Read the model definition and answer for the solid it produces. Units are mm, in the model's axes. Face numbers are marked on the shaded views. A direction names the side the tool comes from. Give positions to 0.01 mm unless a question says otherwise; leave off trailing zeros. Order: outer loops, then holes, each group sorted by start corner. A loop starts at its lowest first (then second) coordinate and runs counter-clockwise, first axis right, second up. Notation, with made-up numbers: (84, 19.25) - (136, 19.25) arc R11 cw to (136, 28.25) - close; hole circle Ø10 at (48.5, 59). An arc over 180 degrees is marked (long way). Use a Markdown table: item, result. Add a question column.
1. Flat-ended cylindrical pins translate along their axes: P1, Ø8, axis at x = -53, z = -9.5, coming from the +Y side; P2, Ø4, axis at x = -22.5, y = 67.5, coming from the +Z side; P3, Ø5, axis at x = -21, y = 29, coming from the +Z side; P4, Ø1.2, axis at y = 86, z = -42.5, coming from the -X side. Find the tip coordinate at first contact, or state that the pin passes through.
2. A cutting plane is placed at A-A on x = -20. Determine the outline of the cut face in (y, z).
3. A cutting plane is placed at B-B on z = 55. Determine the outline of the cut face in (x, y), and give its area (3 significant figures).
4. A cutting plane is placed at C-C on z = -20. Determine the outline of the cut face in (x, y), and give its area (3 significant figures).
5. Consider L1, parallel to X at y = 1, z = 55; L2, parallel to X at y = 100, z = 22; L3, parallel to X at y = 10.5, z = -57. Determine where each line is inside the solid, lowest interval first.
6. Which of the six approach directions +Z, -Z, +X, -X, +Y, -Y give full straight-line access (tool end or side, diameter ignored) to the marked faces 1, 2, 3, 4 and 5?
7. A cutting plane is placed at D-D on y = 44. Determine the outline of the cut face in (x, z).
```python
from build123d import *

# Parameters (mm, degrees)
SKETCH_2_W          = 140
SKETCH_2_H          = 140
EXTRUDE_1_DEPTH     = 4
EXTRUDE_1_2_DEPTH   = 100
EXTRUDE_2_DEPTH     = 2
CUT_EXTRUDE_1_DEPTH = 115.5
SKETCH_6_R          = 6.5
CUT_EXTRUDE_2_DEPTH = 5
FILLET_1_R          = 10
CUT_EXTRUDE_3_REACH = 116


with BuildPart() as part:
    # Эскиз2 → Extrude 1 (new body)
    with BuildSketch(Plane(origin=(0, 0, 0), x_dir=(1, 0, 0), z_dir=(0, 1, 0))):
        Rectangle(SKETCH_2_W, SKETCH_2_H)
    extrude(amount=EXTRUDE_1_DEPTH)

    # Эскиз3 → Extrude 1 2 (add)
    with BuildSketch(Plane(origin=(0, 4, 0), x_dir=(1, 0, 0), z_dir=(0, 1, 0))):
        with BuildLine():
            Line((-40.5, -40), (-40.5, 39))
            ThreePointArc((-40.5, 39), (-40.207106781, 39.707106781), (-39.5, 40))
            Line((-39.5, 40), (39.5, 40))
            ThreePointArc((39.5, 40), (40.207106781, 39.707106781), (40.5, 39))
            Line((40.5, 39), (40.5, -40))
            Line((40.5, -40), (44.5, -40))
            Line((44.5, -40), (44.5, 39))
            ThreePointArc((44.5, 39), (43.035533906, 42.535533906), (39.5, 44))
            Line((39.5, 44), (-39.5, 44))
            ThreePointArc((-39.5, 44), (-43.035533906, 42.535533906), (-44.5, 39))
            Line((-44.5, 39), (-44.5, -40))
            Line((-44.5, -40), (-40.5, -40))
        make_face()
    extrude(amount=EXTRUDE_1_2_DEPTH)

    # Эскиз4 → Бобышка-Вытянуть2 (add, symmetric)
    with BuildSketch(Plane(origin=(0, 0, 0), x_dir=(0, 0, -1), z_dir=(1, 0, 0))):
        Polygon((44, 40.373066959), (65, 4), (44, 4), align=None)
    extrude(amount=EXTRUDE_2_DEPTH, both=True)

    # Эскиз5 → Вырез-Вытянуть1 (cut, through all)
    with BuildSketch(Plane(origin=(44.5, 0, 0), x_dir=(0, 0, -1), z_dir=(1, 0, 0))):
        with BuildLine():
            Line((-15, 92), (-15, 80))
            ThreePointArc((-15, 80), (-20, 75), (-25, 80))
            Line((-25, 80), (-25, 92))
            ThreePointArc((-25, 92), (-20, 97), (-15, 92))
        make_face()
        with BuildLine():
            Line((-15, 28), (-15, 16))
            ThreePointArc((-15, 16), (-20, 11), (-25, 16))
            Line((-25, 16), (-25, 28))
            ThreePointArc((-25, 28), (-20, 33), (-15, 28))
        make_face()
        with BuildLine():
            Line((15, 92), (15, 80))
            ThreePointArc((15, 80), (20, 75), (25, 80))
            Line((25, 80), (25, 92))
            ThreePointArc((25, 92), (20, 97), (15, 92))
        make_face()
        with BuildLine():
            Line((15, 28), (15, 16))
            ThreePointArc((15, 16), (20, 11), (25, 16))
            Line((25, 16), (25, 28))
            ThreePointArc((25, 28), (20, 33), (15, 28))
        make_face()
    extrude(amount=-CUT_EXTRUDE_1_DEPTH, mode=Mode.SUBTRACT)

    # Эскиз6 → Вырез-Вытянуть2 (cut, through all)
    with BuildSketch(Plane(origin=(0, 4, 0), x_dir=(1, 0, 0), z_dir=(0, 1, 0))):
        with Locations(Location((-55, 55, 0), (0, 0, 270))):  # turned: the seam where the file's is
            Circle(SKETCH_6_R)
        with Locations(Location((-55, -55, 0), (0, 0, 270))):  # turned: the seam where the file's is
            Circle(SKETCH_6_R)
        with Locations(Location((55, 55, 0), (0, 0, 270))):  # turned: the seam where the file's is
            Circle(SKETCH_6_R)
        with Locations(Location((55, -55, 0), (0, 0, 270))):  # turned: the seam where the file's is
            Circle(SKETCH_6_R)
    extrude(amount=-CUT_EXTRUDE_2_DEPTH, mode=Mode.SUBTRACT)

    # Скругление1
    fillet_1_edges = [part.edges().sort_by_distance(p)[0] for p in [
        (70, 2, 70),
        (-70, 2, 70),
        (-70, 2, -70),
        (70, 2, -70),
    ]]
    fillet(fillet_1_edges, radius=FILLET_1_R)

    # Эскиз8 → Вырез-Вытянуть3 (cut, up to next)
    with BuildSketch(Plane(origin=(0, 0, -44), x_dir=(-1, 0, 0), z_dir=(0, 0, -1)), mode=Mode.PRIVATE) as cut_extrude_3_sk1:
        with BuildLine():
            Line((-15, 92), (-15, 80))
            ThreePointArc((-15, 80), (-20, 75), (-25, 80))
            Line((-25, 80), (-25, 92))
            ThreePointArc((-25, 92), (-20, 97), (-15, 92))
        make_face()
    cut_extrude_3_tool1 = extrude(cut_extrude_3_sk1.sketch, amount=-CUT_EXTRUDE_3_REACH, mode=Mode.PRIVATE) & part.part
    add(cut_extrude_3_tool1.solids().sort_by_distance((20, 86, -44))[0], mode=Mode.SUBTRACT)
    # Эскиз8 → Вырез-Вытянуть3 (cut, up to next)
    with BuildSketch(Plane(origin=(0, 0, -44), x_dir=(-1, 0, 0), z_dir=(0, 0, -1)), mode=Mode.PRIVATE) as cut_extrude_3_sk2:
        with BuildLine():
            Line((-15, 28), (-15, 16))
            ThreePointArc((-15, 16), (-20, 11), (-25, 16))
            Line((-25, 16), (-25, 28))
            ThreePointArc((-25, 28), (-20, 33), (-15, 28))
        make_face()
    cut_extrude_3_tool2 = extrude(cut_extrude_3_sk2.sketch, amount=-CUT_EXTRUDE_3_REACH, mode=Mode.PRIVATE) & part.part
    add(cut_extrude_3_tool2.solids().sort_by_distance((20, 22, -44))[0], mode=Mode.SUBTRACT)
    # Эскиз8 → Вырез-Вытянуть3 (cut, up to next)
    with BuildSketch(Plane(origin=(0, 0, -44), x_dir=(-1, 0, 0), z_dir=(0, 0, -1)), mode=Mode.PRIVATE) as cut_extrude_3_sk3:
        with BuildLine():
            Line((15, 92), (15, 80))
            ThreePointArc((15, 80), (20, 75), (25, 80))
            Line((25, 80), (25, 92))
            ThreePointArc((25, 92), (20, 97), (15, 92))
        make_face()
    cut_extrude_3_tool3 = extrude(cut_extrude_3_sk3.sketch, amount=-CUT_EXTRUDE_3_REACH, mode=Mode.PRIVATE) & part.part
    add(cut_extrude_3_tool3.solids().sort_by_distance((-20, 86, -44))[0], mode=Mode.SUBTRACT)
    # Эскиз8 → Вырез-Вытянуть3 (cut, up to next)
    with BuildSketch(Plane(origin=(0, 0, -44), x_dir=(-1, 0, 0), z_dir=(0, 0, -1)), mode=Mode.PRIVATE) as cut_extrude_3_sk4:
        with BuildLine():
            Line((15, 28), (15, 16))
            ThreePointArc((15, 16), (20, 11), (25, 16))
            Line((25, 16), (25, 28))
            ThreePointArc((25, 28), (20, 33), (15, 28))
        make_face()
    cut_extrude_3_tool4 = extrude(cut_extrude_3_sk4.sketch, amount=-CUT_EXTRUDE_3_REACH, mode=Mode.PRIVATE) & part.part
    add(cut_extrude_3_tool4.solids().sort_by_distance((-20, 22, -44))[0], mode=Mode.SUBTRACT)


solid = part.part
```
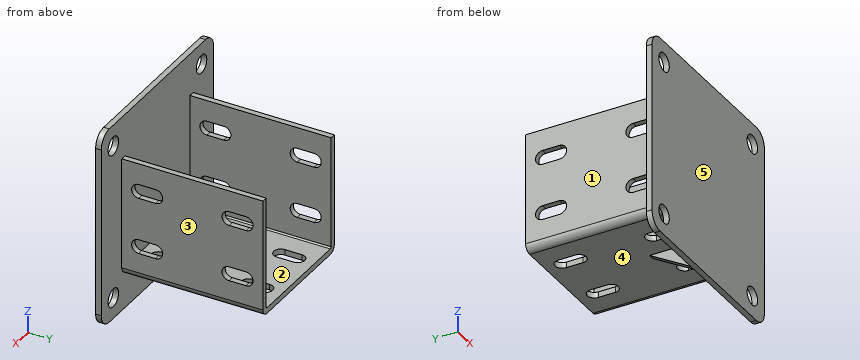
Output values:
| question | item | result |
|---|---|---|
| 1 | P1 | y = 4 |
| 1 | P2 | z = -40 |
| 1 | P3 | through |
| 1 | P4 | x = -43.57 |
| 2 | outline | (0, -70) - (4, -70) - (4, -44) - (11, -44) - (11, -40) - (4, -40) - (4, 70) - (0, 70) - close; (33, -44) - (75, -44) - (75, -40) - (33, -40) - close; (97, -44) - (104, -44) - (104, -40) - (97, -40) - close |
| 3 | outline | (-70, 0) - (-61.5, 0) - (-61.5, 4) - (-70, 4) - close; (-48.5, 0) - (48.5, 0) - (48.5, 4) - (-48.5, 4) - close; (61.5, 0) - (70, 0) - (70, 4) - (61.5, 4) - close |
| 3 | area | 456 mm² |
| 4 | outline | (-70, 0) - (70, 0) - (70, 4) - (44.5, 4) - (44.5, 11) - (40.5, 11) - (40.5, 4) - (-40.5, 4) - (-40.5, 11) - (-44.5, 11) - (-44.5, 4) - (-70, 4) - close; (-44.5, 33) - (-40.5, 33) - (-40.5, 75) - (-44.5, 75) - close; (-44.5, 97) - (-40.5, 97) - (-40.5, 104) - (-44.5, 104) - close; (40.5, 33) - (44.5, 33) - (44.5, 75) - (40.5, 75) - close; (40.5, 97) - (44.5, 97) - (44.5, 104) - (40.5, 104) - close |
| 4 | area | 1,010 mm² |
| 5 | L1 | -70 to -61.5, -48.5 to 48.5, 61.5 to 70 |
| 5 | L2 | -44.5 to -40.5, 40.5 to 44.5 |
| 5 | L3 | -2 to 2 |
| 6 | face 1 | +Z, -Z, -X, +Y |
| 6 | face 2 | +Z, +Y |
| 6 | face 3 | +Z, -Z, +X, +Y |
| 6 | face 4 | -Z, +Y |
| 6 | face 5 | +Z, -Z, +X, -X, -Y |
| 7 | outline | (-44.5, -39) arc R5 ccw to (-39.5, -44) - (39.5, -44) arc R5 ccw to (44.5, -39) - (44.5, 40) - (40.5, 40) - (40.5, -39) arc R1 cw to (39.5, -40) - (-39.5, -40) arc R1 cw to (-40.5, -39) - (-40.5, 40) - (-44.5, 40) - close |
